from build123d import *

# Parameters (mm, degrees)
EXTRUDE1_DEPTH      = 5
SKETCH2_R           = 10
CUT_EXTRUDE1_DEPTH  = 6
BOSS_EXTRUDE1_DEPTH = 40


with BuildPart() as part:
    # Sketch1 → Extrude1 (new body)
    with BuildSketch(Plane.XY):
        with BuildLine():
            Line((0, 40), (0, 0))
            Line((0, 0), (-40, 0))
            Line((-40, 0), (-40, 40))
            ThreePointArc((-40, 40), (-20, 60), (0, 40))
        make_face()
    extrude(amount=EXTRUDE1_DEPTH)

    # Sketch2 → Cut-Extrude1 (cut, through all)
    with BuildSketch(Plane.XY.offset(5)):
        with Locations((-20, 40)):
            Circle(SKETCH2_R)
    extrude(amount=-CUT_EXTRUDE1_DEPTH, mode=Mode.SUBTRACT)

    # Sketch3 → Boss-Extrude1 (add)
    with BuildSketch(Plane(origin=(0, 0, 0), x_dir=(0, 0, -1), z_dir=(1, 0, 0))):
        with BuildLine():
            Line((-10, -5), (-35, -5))
            Line((-35, -5), (-35, -10))
            Line((-35, -10), (-10, -10))
            ThreePointArc((-10, -10), (-2.928932188, -7.071067812), (0, 0))
            Line((0, 0), (-5, 0))
            ThreePointArc((-5, 0), (-6.464466094, -3.535533906), (-10, -5))
        make_face()
    extrude(amount=-BOSS_EXTRUDE1_DEPTH)


solid = part.part
Verification items for the finished model (mm, model axes). A direction names the side the tool comes from. Give positions to 0.01 mm unless a question says otherwise; leave off trailing zeros. Loops run counter-clockwise (first coordinate to the right, second up) from the corner with the lowest first, then second, coordinate; pieces in that order, holes last.
1) Sectioned sample at B-B, the plane y = 41.5. Enter the section's corners in (x, z), then the cut area to 3 significant figures.
2) Thickness scan on line 1 along Y through (x, z) = (-22, 10); line 2 along Z through (x, y) = (-2.5, 8.5); line 3 along Y through (x, z) = (-20, 1.7). Record the ranges inside material, lowest first.
3) Sectioned sample at C-C, the plane y = 7.5. Enter the section's corners in (x, z).
4) Sectioned sample at D-D, the plane z = 21.5. Enter the section's corners in (x, y).
5) Sectioned sample at A-A, the plane x = -20. Enter the section's corners in (y, z).
6) Set-up check for faces 4 (the flat face through (-20, -5, 22)), 5 (the flat face through (-20, -7, 35)): record each of +Z, -Z, +X, -X, +Y, -Y from which the full face is reachable in a straight line by a thin tool's end or side.
7) Draft check along X on faces 1 (the cylindrical face through (-19.72, -7.15, 3.01)), 2 (the cylindrical face through (-20, 60, 2)), 3 (the cylindrical face through (-15.386, 31.128, 2.535)). Enter one of: pulls with the +X half, pulls with the -X half, needs draft (parallel to the pull), parting line crosses it, or undercut.
8) Depth check by flat-ended pin: pin 1 Ø5 at (x, y) = (-6.5, 47) entering from +Z; pin 2 Ø12 at (x, y) = (-20, 40) entering from -Z; pin 3 Ø1 at (x, z) = (-34, 15) entering from +Y. Enter the tip coordinate at first touch or a pass-through.
Answers:
1. outline: (-39.94, 0) - (-29.89, 0) - (-29.89, 5) - (-39.94, 5) - close; (-10.11, 0) - (-0.06, 0) - (-0.06, 5) - (-10.11, 5) - close
1. area: 101 mm2
2. line 1: y = -10 to -5
2. line 2: z = 0 to 5
2. line 3: y = -5.58 to 30, 50 to 60
3. outline: (-40, 0) - (0, 0) - (0, 5) - (-40, 5) - close
4. outline: (-40, -10) - (0, -10) - (0, -5) - (-40, -5) - close
5. outline: (-10, 10) arc R10 ccw to (0, 0) - (30, 0) - (30, 5) - (0, 5) arc R5 cw to (-5, 10) - (-5, 35) - (-10, 35) - close; (50, 0) - (60, 0) - (60, 5) - (50, 5) - close
6. face 4: +Z, +X, -X, +Y
6. face 5: +Z, +X, -X, +Y, -Y
7. face 1: needs draft
7. face 2: parting line crosses it
7. face 3: undercut
8. pin 1: stops at z = 5
8. pin 2: passes through
8. pin 3: stops at y = -5
